from build123d import *

# Parameters (mm, degrees)
SKETCH1_W                = 450
SKETCH1_H                = 350
BOSS_EXTRUDE1_DEPTH      = 20
SKETCH2_R                = 15
CUT_EXTRUDE1_DEPTH       = 25
BOSS_EXTRUDE2_DEPTH      = 10
BOSS_EXTRUDE2_DEPTH_BACK = 30
SKETCH3_R                = 25
SKETCH3_R_2              = 15
FILLET1_R                = 20


with BuildPart() as part:
    # Sketch1 → Boss-Extrude1 (new body)
    with BuildSketch(Plane.XY):
        with Locations((225, -175)):
            Rectangle(SKETCH1_W, SKETCH1_H)
    extrude(amount=BOSS_EXTRUDE1_DEPTH)

    # Sketch2 → Cut-Extrude1 (cut)
    with BuildSketch(Plane(origin=(0, 0, 0), x_dir=(-1, 0, 0), z_dir=(0, 0, -1))):
        with Locations((-420, -175)):
            Circle(SKETCH2_R)
        with Locations((-30, -175)):
            Circle(SKETCH2_R)
    extrude(amount=-CUT_EXTRUDE1_DEPTH, mode=Mode.SUBTRACT)

    # Sketch3 → Boss-Extrude2 (add, two sides: drawn at the far end of the back side and taken through both)
    # profile 1 of 2: a face of its own
    with BuildSketch(Plane(origin=(0, 0, 0), x_dir=(-1, 0, 0), z_dir=(0, 0, -1)).offset(-BOSS_EXTRUDE2_DEPTH_BACK)):
        with Locations((-420, -175)):
            Circle(SKETCH3_R)
        with Locations((-420, -175)):
            Circle(SKETCH3_R_2, mode=Mode.SUBTRACT)
    # profile 2 of 2: a face of its own
    with BuildSketch(Plane(origin=(0, 0, 0), x_dir=(-1, 0, 0), z_dir=(0, 0, -1)).offset(-BOSS_EXTRUDE2_DEPTH_BACK)):
        with Locations((-30, -175)):
            Circle(SKETCH3_R)
        with Locations((-30, -175)):
            Circle(SKETCH3_R_2, mode=Mode.SUBTRACT)
    extrude(amount=BOSS_EXTRUDE2_DEPTH + BOSS_EXTRUDE2_DEPTH_BACK)

    # Fillet1
    fillet1_edges = [part.edges().sort_by_distance(p)[0] for p in [
        (0, 0, 10),
        (450, 0, 10),
        (450, -350, 10),
        (0, -350, 10),
    ]]
    fillet(fillet1_edges, radius=FILLET1_R)


solid = part.part
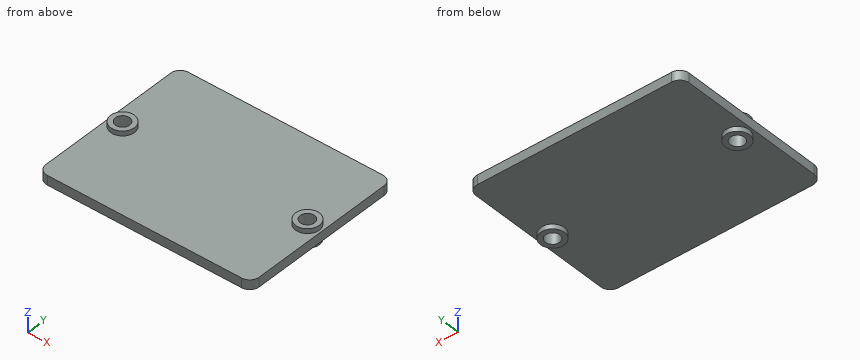
Read the model definition and answer for the solid it produces. Units are mm, in the model's axes. Round coordinates to 2 decimals unless told otherwise and drop trailing zeros. Order: outer loops, then holes, each group sorted by start corner. A loop starts at its lowest first (then second) coordinate and runs counter-clockwise, first axis right, second up. Notation, with made-up numbers: (12.5, 46.25) - (38.5, 46.25) arc R35 cw to (38.5, 80.25) - close; hole circle Ø10 at (76.25, 54.5). An arc over 180 degrees is marked (long way). Use one line per item in the form item = value. Start each with the question number.
(1) The part is cut by section A-A (y = -175). Give the vertices of the cut face in (x, z), then the cut area to 3 significant figures.
(2) The part is cut by section B-B (x = 30). Give the vertices of the cut face in (y, z).
(3) The part is cut by section C-C (x = 83). Give the vertices of the cut face in (y, z), then the cut area to 3 significant figures.
(4) Find the intervals of material crossed by line 1 along Y through (x, z) = (30, 10); line 2 along Y through (x, z) = (30, -1); line 3 along Z through (x, y) = (144.5, -306), in increasing order. Write a range as from..to.
(5) The part is cut by section D-D (y = -252.5). Give the vertices of the cut face in (x, z), then the cut area to 3 significant figures.
(6) Flat-ended cylindrical pins translate along their axes: pin 1 Ø6 at (x, y) = (163.5, -141) entering from -Z; pin 2 Ø2 at (x, y) = (50.5, -283.5) entering from +Z. Find the tip coordinate at first contact, or state that the pin passes through.
Checked values:
q1.outline = (0, 0) - (5, 0) - (5, -10) - (15, -10) - (15, 30) - (5, 30) - (5, 20) - (0, 20) - close; (45, -10) - (55, -10) - (55, 0) - (395, 0) - (395, -10) - (405, -10) - (405, 30) - (395, 30) - (395, 20) - (55, 20) - (55, 30) - (45, 30) - close; (435, -10) - (445, -10) - (445, 0) - (450, 0) - (450, 20) - (445, 20) - (445, 30) - (435, 30) - close
q1.area = 8,600 mm^2
q2.outline = (-350, 0) - (-200, 0) - (-200, -10) - (-190, -10) - (-190, 30) - (-200, 30) - (-200, 20) - (-350, 20) - close; (-160, -10) - (-150, -10) - (-150, 0) - (0, 0) - (0, 20) - (-150, 20) - (-150, 30) - (-160, 30) - close
q3.outline = (-350, 0) - (0, 0) - (0, 20) - (-350, 20) - close
q3.area = 7,000 mm^2
q4.line_1 = -350..-190, -160..0
q4.line_2 = -200..-190, -160..-150
q4.line_3 = 0..20
q5.outline = (0, 0) - (450, 0) - (450, 20) - (0, 20) - close
q5.area = 9,000 mm^2
q6.pin_1 = 0
q6.pin_2 = 20
